Read the model definition and answer for the solid it produces. Units are mm, in the model's axes. A direction names the side the tool comes from. Coordinates: 2 decimals unless noted, no trailing zeros. Loops run counter-clockwise (first coordinate to the right, second up) from the corner with the lowest first, then second, coordinate; pieces in that order, holes last. Notation, with made-up numbers: (-17.5, 55) - (-4.5, 55) arc R17 cw to (-4.5, 63) - close; hole circle Ø1 at (-21, 60). An arc over 180 degrees is marked (long way). Use one line per item in the form item = value.
Solid Edge part; units mm, degrees
sketch "Sketch1" plane through (0, 0, 0) normal (0, -1, 0) x (1, 0, 0)
  line L0 (30, 9) -> (67.1942, -9.0603)
  arc A0 (67.3406, -9.1875) -> (98.8277, -9.1875) centre (83.0842, 9.0978) ccw
  arc A1 (98.8277, -9.1875) -> (102.5044, -11.2909) centre (100.2937, -10.8901) cw
  arc A2 (72.6505, -17.0171) -> (102.5044, -11.2909) centre (83.092, 9.2313) ccw
  line L1 (72.6237, -17.0064) -> (30, 0)
  line L2 (30, 0) -> (0, 0)
  line L3 (0, 0) -> (0, 9)
  line L4 (0, 9) -> (30, 9)
  arc A3 (67.3406, -9.1875) -> (67.1942, -9.0603) centre (83, 9) cw
  arc A4 (72.6505, -17.0171) -> (72.6237, -17.0064) centre (83, 9) cw
extrude "Protrusion1" add sketch "Sketch1" against normal blind 30
sketch "Sketch2" plane through (48.5971, 15, -0.0302) normal (0.4367982, 0, 0.8995595) x (0, 1, 0)
  line L0 (-10, 20.6735) -> (-10, -53.4115)
  line L1 (0, 20.6735) -> (-10, 20.6735)
  line L2 (0, 20.6735) -> (10, 20.6735)
  line L3 (10, 20.6735) -> (10, -53.4115)
extrude "Recorte_Extrudado_1" cut sketch "Sketch2" along normal blind 140 material side at (63.322, 5.05, -7.1801)
sketch "Sketch3" plane through (48.5971, 15, -0.0302) normal (0.4367982, 0, 0.8995595) x (0, 1, 0)
  line L0 (10, 20.6735) -> (10, -53.4115)
  line L1 (0, 20.6735) -> (10, 20.6735)
  line L2 (0, 20.6735) -> (-10, 20.6735)
  line L3 (-10, 20.6735) -> (-10, -53.4115)
extrude "Recorte_Extrudado_2" cut sketch "Sketch3" against normal blind 100 material side at (63.322, 24.95, -7.1801)
fillet "Redondo_1" radius 2 3 edges at (27.8149, 5, 4.5) (0, 0, 4.5) (0, 30, 4.5)
fillet "Redondo_1" radius 1 1 edges at (27.8149, 25, 4.5)
sketch "Sketch4" plane through (0, 0, 0) normal (0, -1, 0) x (1, 0, 0)
  circle A0 centre (15, 4.5) radius 2.5
extrude "Recorte_Extrudado_3" cut sketch "Sketch4" against normal blind 100
fillet "Redondo_3" radius 1 12 edges at (51.3119, 30, -8.5032) (72.6371, 30, -17.0117) (88.4133, 30, -18.5119) (51.3119, 25, -8.5032) (72.6371, 25, -17.0117) (88.4133, 25, -18.5119) (51.3119, 5, -8.5032) (72.6371, 5, -17.0117) (88.4133, 5, -18.5119) (51.3119, 0, -8.5032) (72.6371, 0, -17.0117) (88.4133, 0, -18.5119)
Item 1: Which of the six approach directions +Z, -Z, +X, -X, +Y, -Y give full straight-line access (tool end or side, diameter ignored) to faces 5 (the cylindrical face through (88.193, 27.479, -18.553)), 6 (the cylindrical face through (51.72, 4.7, -8.36)), 7 (the cylindrical face through (28.325, 5.57, 4.174))?
Results below:
face_5 = -Z, +Y, -Y
face_6 = -Z, -X
face_7 = -Z, +X
Item 2: For a pull along Y with two mould halves and no side action, classify faces 1 (the cylindrical face through (28.04, 24.7, 4.31)), 2 (the flat face through (41, 0, -3)), 3 (the cylindrical face through (12.5, 14.8, 4.6)), 4 (the flat face through (41, 30, -3)) as +Y half, -Y half, draft (parallel to the pull), parting line (faces both ways), or undercut.
Results below:
face_1 = undercut
face_2 = -Y half
face_3 = draft
face_4 = +Y half
Item 3: Find the intervals of material crossed by L1, parallel to Z at x = 15, y = 19.75; L2, parallel to Y at x = 57.5, z = -7; L3, parallel to Z at x = 25.5, y = 15.5, in increasing order.
Results below:
L1 = 0 to 2, 7 to 9
L2 = 0 to 5, 25 to 30
L3 = 0 to 9
Item 4: Each of these flat-tipped pins is pushed along its axis until it touches: P1, Ø8, axis at x = 68.5, z = -4, coming from the -Y side; P2, Ø12, axis at x = 14, y = 13, coming from the -Z side. Where does it stop, or does it pass through?
Results below:
P1 = through
P2 = 0
Item 5: The part is cut by section B-B on z = -12.25. Count the separate pieces of the cut face and the enclosed holes in it, plus the area to 3 significant figures.
Results below:
separate_pieces = 4
enclosed_holes = 0
area = 179 mm²
Item 6: The part is cut by section A-A on x = 15. Give the vertices of the cut face in (y, z).
Results below:
outline = (0, 0) - (30, 0) - (30, 2) - (0, 2) - close; (0, 7) - (30, 7) - (30, 9) - (0, 9) - close
